from build123d import *

# Parameters (mm, degrees)
SKETCH1_W             = 76
SKETCH1_H             = 62
BOSS_EXTRUDE1_DEPTH   = 2
SKETCH2_W             = 82
SKETCH2_H             = 68
BOSS_EXTRUDE2_DEPTH   = 8
SKETCH3_W             = 60
SKETCH3_H             = 12.8
CUT_EXTRUDE1_DEPTH    = 11
SKETCH4_R             = 1.6
CUT_EXTRUDE2_DEPTH    = 11
SKETCH5_R             = 3.1
CUT_EXTRUDE3_DEPTH    = 3
SKETCH9_OUTSIDE_W     = 105.4
SKETCH9_OUTSIDE_H     = 91.4
SKETCH9_OUTSIDE_W_2   = 75.6
SKETCH9_OUTSIDE_H_2   = 61.6
CUT_EXTRUDE5_DEPTH    = 3
CUT_EXTRUDE6_DEPTH    = 3
SKETCH11_W            = 66
SKETCH11_H            = 54
CUT_EXTRUDE7_DEPTH    = 7
CHAMFER2_SIZE         = 2
CHAMFER2_SIZE2        = 0.352653961
CHAMFER2_PART_2_SIZE  = 2
CHAMFER2_PART_2_SIZE2 = 0.352653961
CHAMFER3_SIZE         = 1
CHAMFER3_SIZE2        = 1.732050808


with BuildPart() as part:
    # Sketch1 → Boss-Extrude1 (new body)
    with BuildSketch(Plane(origin=(0, 0, 0), x_dir=(1, 0, 0), z_dir=(0, 1, 0))):
        Rectangle(SKETCH1_W, SKETCH1_H)
    extrude(amount=BOSS_EXTRUDE1_DEPTH)

    # Sketch2 → Boss-Extrude2 (add)
    with BuildSketch(Plane(origin=(0, 2, 0), x_dir=(1, 0, 0), z_dir=(0, 1, 0))):
        Rectangle(SKETCH2_W, SKETCH2_H)
    extrude(amount=BOSS_EXTRUDE2_DEPTH)

    # Sketch3 → Cut-Extrude1 (cut, through all)
    with BuildSketch(Plane.XZ):
        with Locations((0, -12.5)):
            Rectangle(SKETCH3_W, SKETCH3_H)
        with Locations((0, 12.5)):
            Rectangle(SKETCH3_W, SKETCH3_H)
    extrude(amount=-CUT_EXTRUDE1_DEPTH, mode=Mode.SUBTRACT)

    # Sketch4 → Cut-Extrude2 (cut, through all)
    with BuildSketch(Plane(origin=(0, 10, 0), x_dir=(1, 0, 0), z_dir=(0, 1, 0))):
        with Locations(Location((-35.408866178, 29.363450001, 0), (0, 0, 270))):  # turned: the seam where the file's is
            Circle(SKETCH4_R)
        with Locations(Location((35.408866178, 29.363450001, 0), (0, 0, 270))):  # turned: the seam where the file's is
            Circle(SKETCH4_R)
        with Locations(Location((35.408866178, -29.363450001, 0), (0, 0, 270))):  # turned: the seam where the file's is
            Circle(SKETCH4_R)
        with Locations(Location((-35.408866178, -29.363450001, 0), (0, 0, 270))):  # turned: the seam where the file's is
            Circle(SKETCH4_R)
    extrude(amount=-CUT_EXTRUDE2_DEPTH, mode=Mode.SUBTRACT)

    # Sketch5 → Cut-Extrude3 (cut)
    with BuildSketch(Plane(origin=(0, 10, 0), x_dir=(1, 0, 0), z_dir=(0, 1, 0))):
        with Locations(Location((-35.408866178, 29.363450001, 0), (0, 0, 270))):  # turned: the seam where the file's is
            Circle(SKETCH5_R)
        with Locations(Location((35.408866178, 29.363450001, 0), (0, 0, 270))):  # turned: the seam where the file's is
            Circle(SKETCH5_R)
        with Locations(Location((35.408866178, -29.363450001, 0), (0, 0, 270))):  # turned: the seam where the file's is
            Circle(SKETCH5_R)
        with Locations(Location((-35.408866178, -29.363450001, 0), (0, 0, 270))):  # turned: the seam where the file's is
            Circle(SKETCH5_R)
    extrude(amount=-CUT_EXTRUDE3_DEPTH, mode=Mode.SUBTRACT)

    # Sketch9 outside → Cut-Extrude5 (cut)
    with BuildSketch(Plane.XZ):
        Rectangle(SKETCH9_OUTSIDE_W, SKETCH9_OUTSIDE_H)
        Rectangle(SKETCH9_OUTSIDE_W_2, SKETCH9_OUTSIDE_H_2, mode=Mode.SUBTRACT)
    extrude(amount=-CUT_EXTRUDE5_DEPTH, mode=Mode.SUBTRACT)

    # Sketch10 → Cut-Extrude6 (cut)
    with BuildSketch(Plane.XZ):
        Polygon((-37.8, -30.8), (-31.8, -30.8), (-37.8, -24.8), align=None)
        Polygon((-37.8, 24.8), (-37.8, 30.8), (-31.8, 30.8), align=None)
        Polygon((37.8, 30.8), (37.8, 24.8), (31.8, 30.8), align=None)
        Polygon((37.8, -30.8), (31.8, -30.8), (37.8, -24.8), align=None)
    extrude(amount=-CUT_EXTRUDE6_DEPTH, mode=Mode.SUBTRACT)

    # Sketch11 → Cut-Extrude7 (cut)
    with BuildSketch(Plane.XZ):
        Rectangle(SKETCH11_W, SKETCH11_H)
    extrude(amount=-CUT_EXTRUDE7_DEPTH, mode=Mode.SUBTRACT)

    # Chamfer2
    chamfer2_edges = [part.edges().sort_by_distance(p)[0] for p in [
        (37.8, 0, 0),
    ]]
    chamfer2_side = [part.faces().sort_by_distance(p)[0] for p in [
        (37.8, 1.5, 0),
    ]]
    chamfer(chamfer2_edges, length=CHAMFER2_SIZE, length2=CHAMFER2_SIZE2, reference=chamfer2_side[0])

    # Chamfer2 part 2
    chamfer2_part_2_edges = [part.edges().sort_by_distance(p)[0] for p in [
        (-37.8, 0, 0),
    ]]
    chamfer2_part_2_side = [part.faces().sort_by_distance(p)[0] for p in [
        (-37.8, 1.5, 0),
    ]]
    chamfer(chamfer2_part_2_edges, length=CHAMFER2_PART_2_SIZE, length2=CHAMFER2_PART_2_SIZE2, reference=chamfer2_part_2_side[0])

    # Chamfer3
    chamfer3_edges = [part.edges().sort_by_distance(p)[0] for p in [
        (0, 0, -30.8),
        (0, 0, 30.8),
    ]]
    chamfer3_side = [part.faces().sort_by_distance(p)[0] for p in [
        (-35.357643735, 0, 25.870950059),
    ]]
    chamfer(chamfer3_edges, length=CHAMFER3_SIZE, length2=CHAMFER3_SIZE2, reference=chamfer3_side[0])


solid = part.part
The listing builds one solid part. Answer for the finished solid, in the listing's coordinates (mm). A direction names the side the tool comes from. Coordinates: 2 decimals unless noted, no trailing zeros. Order: outer loops, then holes, each group sorted by start corner. A loop starts at its lowest first (then second) coordinate and runs counter-clockwise, first axis right, second up. Notation, with made-up numbers: (59, 33.5) -> (67, 33.5) arc R9 ccw to (67, 47.5) -> close; hole circle Ø11 at (40, 50.25). An arc over 180 degrees is marked (long way). Answer in a Markdown table with one row per item. Add a question column.
Item 1: Find section A-A (z = -10). Write down the section's boundary in (x, y), then the cut area to 3 significant figures.
Item 2: Which of the six approach directions +Z, -Z, +X, -X, +Y, -Y give full straight-line access (tool end or side, diameter ignored) to faces 1 (the face through (-36.2, 1.5, 26.4)), 2 (the face through (36.2, 1.5, -26.4)), 3 (the face through (-37, 7, -28)), 4 (the face through (-36.2, 1.5, -26.4))?
Item 3: Find section B-B (x = 8.5). Write down the section's boundary in (y, z), then the cut area to 3 significant figures.
Item 4: Find the intervals of material crossed by L1, parallel to Z at x = 23.5, y = 8.25; L2, parallel to X at y = 9, z = 29; L3, parallel to Z at x = -24, y = 4.5, in increasing order. Write a range as from..to.
Item 5: Each of these flat-tipped pins is pushed along its axis until it touches: P1, Ø10, axis at x = -6, z = 17, coming from the -Y side; P2, Ø1.5, axis at y = 2, z = -27, coming from the -X side; P3, Ø1.9, axis at x = -35.41, z = 29.36, coming from the +Y side; P4, Ø0.8, axis at y = 2.5, z = 5, coming from the +X side. Where does it stop, or does it pass through?
Item 6: Find section C-C (y = 8). Write down the section's boundary in (x, z).
Item 7: Determine the mould class of faces 5 (the face through (0, 3, 27)), 6 (the face through (-37, 7, 31)), 7 (the face through (-37.62, 0.99, -0.35)), 8 (the face through (32.9, 1.5, -29.7)) for opening direction Z: +Z half, -Z half, draft (parallel to the pull), parting line (faces both ways), or undercut.
Item 8: Find section D-D (z = 3.5). Write down the section's boundary in (x, y).
Result set:
| question | item | result |
|---|---|---|
| 1 | outline | (-41, 3) -> (-37.8, 3) -> (-37.8, 2) -> (-37.45, 0) -> (-33, 0) -> (-33, 7) -> (-30, 7) -> (-30, 10) -> (-41, 10) -> close; (30, 7) -> (33, 7) -> (33, 0) -> (37.45, 0) -> (37.8, 2) -> (37.8, 3) -> (41, 3) -> (41, 10) -> (30, 10) -> close |
| 1 | area | 158 mm² |
| 2 | face 1 | +Z, -X, -Y |
| 2 | face 2 | -Z, +X, -Y |
| 2 | face 3 | +Y |
| 2 | face 4 | -Z, -X, -Y |
| 3 | outline | (0, -29.8) -> (1.73, -30.8) -> (3, -30.8) -> (3, -34) -> (10, -34) -> (10, -18.9) -> (7, -18.9) -> (7, -27) -> (0, -27) -> close; (0, 27) -> (7, 27) -> (7, 18.9) -> (10, 18.9) -> (10, 34) -> (3, 34) -> (3, 30.8) -> (1.73, 30.8) -> (0, 29.8) -> close; (7, -6.1) -> (10, -6.1) -> (10, 6.1) -> (7, 6.1) -> close |
| 3 | area | 204 mm² |
| 4 | L1 | z = -34..-18.9, -6.1..6.1, 18.9..34 |
| 4 | L2 | x = -41..-38.49, -32.33..32.33, 38.49..41 |
| 4 | L3 | z = -34..-27, 27..34 |
| 5 | P1 | stops at y = 7 |
| 5 | P2 | stops at x = -36.35 |
| 5 | P3 | passes through |
| 5 | P4 | stops at x = 37.8 |
| 6 | outline | (-41, -34) -> (41, -34) -> (41, 34) -> (-41, 34) -> close; hole circle Ø6.2 at (-35.41, -29.36); hole circle Ø6.2 at (-35.41, 29.36); hole (-30, -18.9) -> (30, -18.9) -> (30, -6.1) -> (-30, -6.1) -> close; hole (-30, 6.1) -> (30, 6.1) -> (30, 18.9) -> (-30, 18.9) -> close; hole circle Ø6.2 at (35.41, -29.36); hole circle Ø6.2 at (35.41, 29.36) |
| 7 | face 5 | undercut |
| 7 | face 6 | undercut |
| 7 | face 7 | draft |
| 7 | face 8 | -Z half |
| 8 | outline | (-41, 3) -> (-37.8, 3) -> (-37.8, 2) -> (-37.45, 0) -> (-33, 0) -> (-33, 7) -> (33, 7) -> (33, 0) -> (37.45, 0) -> (37.8, 2) -> (37.8, 3) -> (41, 3) -> (41, 10) -> (-41, 10) -> close |
